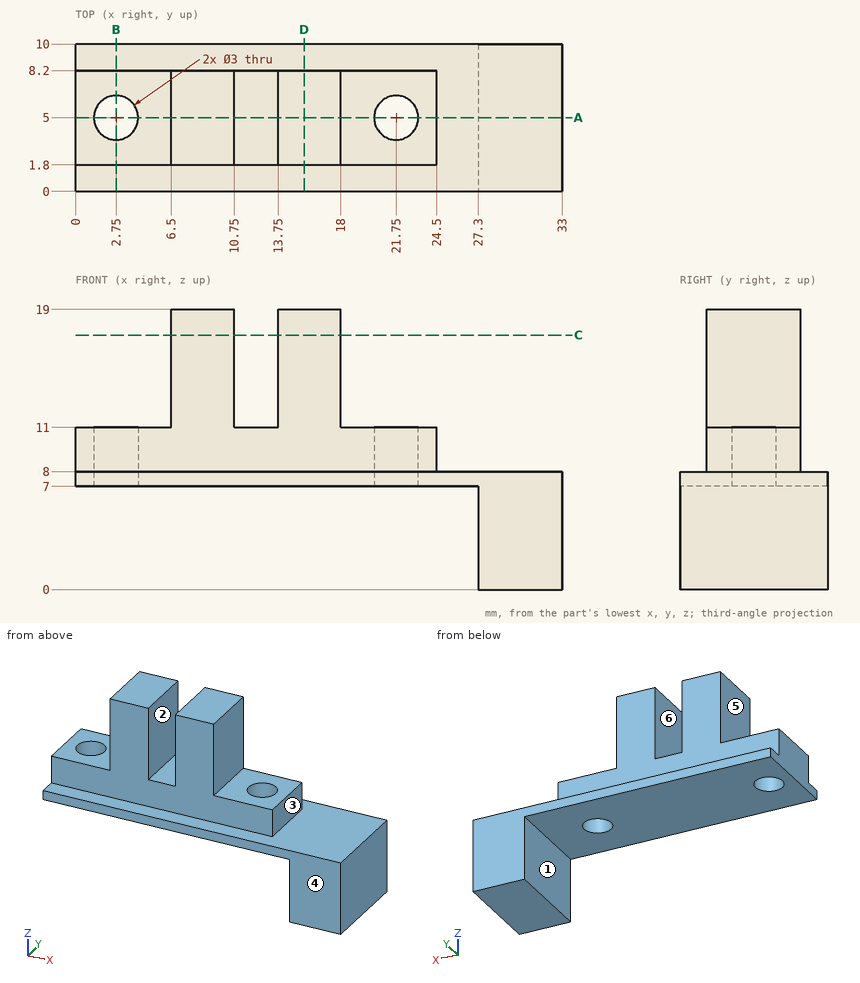
Check sheet for the drawn part. Datum: minimum x, y, z corner. Units: mm. A direction names the side the tool comes from. Give positions to 0.01 mm unless a question says otherwise; leave off trailing zeros. Order: outer loops, then holes, each group sorted by start corner. A loop starts at its lowest first (then second) coordinate and runs counter-clockwise, first axis right, second up. Notation, with made-up numbers: (89.25, -12.75) -> (140.25, -12.75) arc R5 ccw to (140.25, -5.75) -> close; hole circle Ø3 at (63.5, 27). An arc over 180 degrees is marked (long way). Use a Markdown table: item, result.
1) Section check D-D, the plane x = 15.5. Record the boundary of the cut face in (y, z).
Results:
| item | result |
|---|---|
| outline | (0, 7) -> (10, 7) -> (10, 8) -> (8.2, 8) -> (8.2, 19) -> (1.8, 19) -> (1.8, 8) -> (0, 8) -> close |
2) Mould release check, pull along X, two halves, no side actions. Record for the marked faces 4, 5 and 6: pulls with the +X half, pulls with the -X half, needs draft (parallel to the pull), parting line crosses it, or undercut.
Results:
| item | result |
|---|---|
| face 4 | needs draft |
| face 5 | pulls with the -X half |
| face 6 | undercut |
3) Tool access check on the marked faces 1, 2 and 3. Record the directions out of +Z, -Z, +X, -X, +Y, -Y that give a thin tool (end or side, any length) a straight path to the whole face; none if there is none.
Results:
| item | result |
|---|---|
| face 1 | -Z, -X, +Y, -Y |
| face 2 | +Z, +Y, -Y |
| face 3 | +Z, +X, +Y, -Y |
4) Section check C-C, the plane z = 17.25. Record the boundary of the cut face in (x, y), then the cut area to 3 significant figures.
Results:
| item | result |
|---|---|
| outline | (6.5, 1.8) -> (10.75, 1.8) -> (10.75, 8.2) -> (6.5, 8.2) -> close; (13.75, 1.8) -> (18, 1.8) -> (18, 8.2) -> (13.75, 8.2) -> close |
| area | 54.4 mm² |
5) Section check B-B, the plane x = 2.75. Record the boundary of the cut face in (y, z).
Results:
| item | result |
|---|---|
| outline | (0, 7) -> (3.5, 7) -> (3.5, 11) -> (1.8, 11) -> (1.8, 8) -> (0, 8) -> close; (6.5, 7) -> (10, 7) -> (10, 8) -> (8.2, 8) -> (8.2, 11) -> (6.5, 11) -> close |
6) Depth check by flat-ended pin: pin 1 Ø1.9 at (y, z) = (4, 15.5) entering from +X; pin 2 Ø3.5 at (y, z) = (4, 4) entering from -X; pin 3 Ø1.5 at (y, z) = (6, 9) entering from +X. Enter the tip coordinate at first touch or a pass-through.
Results:
| item | result |
|---|---|
| pin 1 | x = 18 |
| pin 2 | x = 27.3 |
| pin 3 | x = 24.5 |
7) Section check A-A, the plane y = 5. Record the boundary of the cut face in (x, z), then the cut area to 3 significant figures.
Results:
| item | result |
|---|---|
| outline | (0, 7) -> (1.25, 7) -> (1.25, 11) -> (0, 11) -> close; (4.25, 7) -> (20.25, 7) -> (20.25, 11) -> (18, 11) -> (18, 19) -> (13.75, 19) -> (13.75, 11) -> (10.75, 11) -> (10.75, 19) -> (6.5, 19) -> (6.5, 11) -> (4.25, 11) -> close; (23.25, 7) -> (27.3, 7) -> (27.3, 0) -> (33, 0) -> (33, 8) -> (24.5, 8) -> (24.5, 11) -> (23.25, 11) -> close |
| area | 190 mm² |
8) Material ranges on probe 1 along Y at (x, z) = (21.75, 8.65); probe 2 along X at (y, z) = (5, 15); probe 3 along Z at (x, y) = (6, 3), recorded low to high.
Results:
| item | result |
|---|---|
| probe 1 | 1.8 to 3.5, 6.5 to 8.2 |
| probe 2 | 6.5 to 10.75, 13.75 to 18 |
| probe 3 | 7 to 11 |
